```python
from build123d import *

# Parameters (mm, degrees)
SKETCH1_W           = 10.922
SKETCH1_H           = 8.128
BOSS_EXTRUDE1_DEPTH = 0.635
CHAMFER1_SIZE       = 0.635


with BuildPart() as part:
    # Sketch1 → Boss-Extrude1 (new body)
    with BuildSketch(Plane(origin=(0, 0, 0), x_dir=(1, 0, 0), z_dir=(0, 1, 0))):
        Rectangle(SKETCH1_W, SKETCH1_H)
    extrude(amount=BOSS_EXTRUDE1_DEPTH)

    # Chamfer1
    chamfer1_edges = [part.edges().sort_by_distance(p)[0] for p in [
        (0, 0.635, 4.064),
    ]]
    chamfer(chamfer1_edges, length=CHAMFER1_SIZE - 0.0001)  # a hair under: the kernel refuses the full size


solid = part.part
```
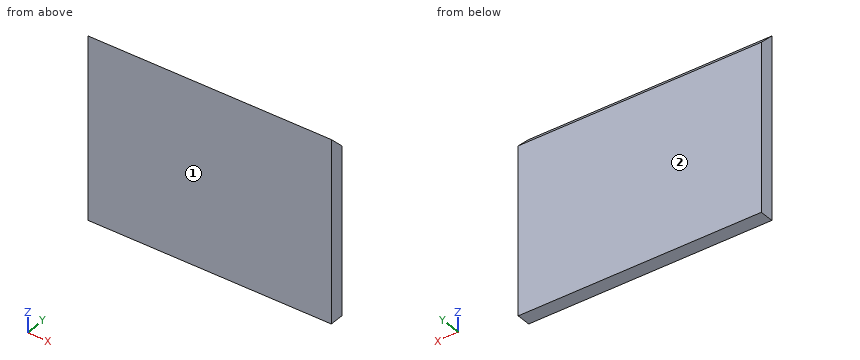
Work out the finished part from the listing and answer in its coordinate system (mm). Face numbers are marked on the shaded views. Give positions to 0.01 mm unless a question says otherwise; leave off trailing zeros. Write each loop counter-clockwise with the first axis right and the second up, starting at its lowest first coordinate (ties: lowest second). Pieces come first, ordered by that corner, then holes.
(1) The mould has two halves that part along Y. Classify the marked faces 1 and 2: pulls with the +Y half, pulls with the -Y half, needs draft (parallel to the pull), parting line crosses it, or undercut.
Final values:
face 1: pulls with the -Y half
face 2: pulls with the +Y half
(2) Straight lines are drawn through the part: line 1 (Z direction, x = 2.5, y = 0.4); line 2 (Z direction, x = 2.25, y = 0.3). For each, find the intervals that lie inside material, in ascending order.
Final values:
line 1: z = -4.06 to 3.66
line 2: z = -4.06 to 3.76
(3) The part is cut by section B-B on y = 0.3. Write down the section's boundary in (x, z), plus the area to 3 significant figures.
Final values:
outline: (-5.46, -4.06) - (5.46, -4.06) - (5.46, 3.76) - (-5.46, 3.76) - close
area: 85.5 mm2
